from build123d import *

# Parameters (mm, degrees)
SKETCH1_W                                      = 34
SKETCH1_H                                      = 2.5
EXTRUDE1_DEPTH                                 = 38.5
FILLET1_R                                      = 2
SKETCH2_W                                      = 31.6
SKETCH2_H                                      = 36.1
EXTRUDE2_DEPTH                                 = 1
CSK_FOR_1_FLAT_HEAD_MACHINE_SCREW1_D           = 2.0574
CSK_FOR_1_FLAT_HEAD_MACHINE_SCREW1_CSINK_D     = 3.7084
CSK_FOR_1_FLAT_HEAD_MACHINE_SCREW1_CSINK_ANGLE = 82


with BuildPart() as part:
    # Sketch1 → Extrude1 (new body)
    with BuildSketch(Plane.XY):
        with Locations((-7.05, 3.25)):
            Rectangle(SKETCH1_W, SKETCH1_H)
    extrude(amount=-EXTRUDE1_DEPTH)

    # Fillet1
    fillet1_edges = [part.edges().sort_by_distance(p)[0] for p in [
        (9.95, 3.25, -38.5),
        (9.95, 3.25, 0),
        (-24.05, 3.25, 0),
        (-24.05, 3.25, -38.5),
    ]]
    fillet(fillet1_edges, radius=FILLET1_R)

    # Sketch2 → Extrude2 (add)
    with BuildSketch(Plane.XZ.offset(-2)):
        with Locations((-7.05, -19.25)):
            Rectangle(SKETCH2_W, SKETCH2_H)
    extrude(amount=EXTRUDE2_DEPTH)

    # CSK for #1 Flat Head Machine Screw1 (through all)
    with Locations(Plane(origin=(-20.25, 4.5, -34.7), x_dir=(0, 0, 1), z_dir=(0, 1, 0))):
        with Locations((0, 0)):
            CounterSinkHole(CSK_FOR_1_FLAT_HEAD_MACHINE_SCREW1_D / 2, CSK_FOR_1_FLAT_HEAD_MACHINE_SCREW1_CSINK_D / 2, counter_sink_angle=CSK_FOR_1_FLAT_HEAD_MACHINE_SCREW1_CSINK_ANGLE)


solid = part.part
The listing builds one solid part. Answer for the finished solid, in the listing's coordinates (mm). A direction names the side the tool comes from. Round coordinates to 2 decimals unless told otherwise and drop trailing zeros. Write each loop counter-clockwise with the first axis right and the second up, starting at its lowest first coordinate (ties: lowest second). Pieces come first, ordered by that corner, then holes. Notation, with made-up numbers: (26.5, -8) - (84.5, -8) arc R17 cw to (84.5, -4) - close; hole circle Ø8 at (6.25, -4.75). An arc over 180 degrees is marked (long way). Use one line per item in the form item = value. Start each with the question number.
Item 1: A cutting plane is placed at D-D (x = -6). Write down the section's boundary in (y, z).
Item 2: A cutting plane is placed at A-A (z = -34.7). Write down the section's boundary in (x, y).
Item 3: A cutting plane is placed at C-C (y = 1.55). Write down the section's boundary in (x, z).
Item 4: Find the intervals of material crossed by line 1 (X direction, y = 2.05, z = -34.7); line 2 (Z direction, x = -20.25, y = 1.7); line 3 (X direction, y = 1.9, z = -34.7), in increasing order. Write a range as [from, to].
Item 5: A tool of negligible diameter and unlimited length cuts with its end or side. For faces 4 (the flat face through (-7, 4.5, -19)), 5 (the flat face through (9.95, 3, -19)), 6 (the flat face through (8.75, 1.5, -19.5)), 7 (the flat face through (-22.85, 1.5, -19.5)), 8 (the flat face through (-7.3, 1.5, -37.3)), from which of +Z, -Z, +X, -X, +Y, -Y can it reach the whole face along a straight path? Write none if from no direction.
Item 6: A cutting plane is placed at B-B (x = -20.25). Write down the section's boundary in (y, z), plus the area to 3 significant figures.
Item 7: Flat-ended cylindrical pins translate along their axes: pin 1 Ø0.8 at (y, z) = (1.5, -16.5) entering from -X; pin 2 Ø0.8 at (x, y) = (-0.5, 1.5) entering from +Z. Find the tip coordinate at first contact, or state that the pin passes through.
Item 8: Determine the mould class of faces 1 (the flat face through (-7.3, 1.5, -1.2)), 2 (the flat face through (-7, 3, -38.5)), 3 (the cylindrical face through (-21.254, 2.257, -34.477)) for opening direction Z: +Z half, -Z half, draft (parallel to the pull), parting line (faces both ways), or undercut.
The answers:
q1.outline = (1, -37.3) - (2, -37.3) - (2, -38.5) - (4.5, -38.5) - (4.5, 0) - (2, 0) - (2, -1.2) - (1, -1.2) - close
q2.outline = (-24.05, 2) - (-22.85, 2) - (-22.85, 1) - (-21.28, 1) - (-21.28, 3.55) - (-22.1, 4.5) - (-24.05, 4.5) - close; (-19.22, 1) - (8.75, 1) - (8.75, 2) - (9.95, 2) - (9.95, 4.5) - (-18.4, 4.5) - (-19.22, 3.55) - close
q3.outline = (-22.85, -37.3) - (8.75, -37.3) - (8.75, -1.2) - (-22.85, -1.2) - close; hole circle Ø2.06 at (-20.25, -34.7)
q4.line_1 = [-24.05, -21.28], [-19.22, 9.95]
q4.line_2 = [-37.3, -35.73], [-33.67, -1.2]
q4.line_3 = [-22.85, -21.28], [-19.22, 8.75]
q5.face_4 = +Z, -Z, +X, -X, +Y
q5.face_5 = +Z, -Z, +X, +Y, -Y
q5.face_6 = +Z, -Z, +X, -Y
q5.face_7 = +Z, -Z, -X, -Y
q5.face_8 = -Z, +X, -X, -Y
q6.outline = (1, -37.3) - (2, -37.3) - (2, -38.5) - (4.5, -38.5) - (4.5, -36.55) - (3.55, -35.73) - (1, -35.73) - close; (1, -33.67) - (3.55, -33.67) - (4.5, -32.85) - (4.5, 0) - (2, 0) - (2, -1.2) - (1, -1.2) - close
q6.area = 124 mm^2
q7.pin_1 = -22.85
q7.pin_2 = -1.2
q8.face_1 = +Z half
q8.face_2 = -Z half
q8.face_3 = undercut
